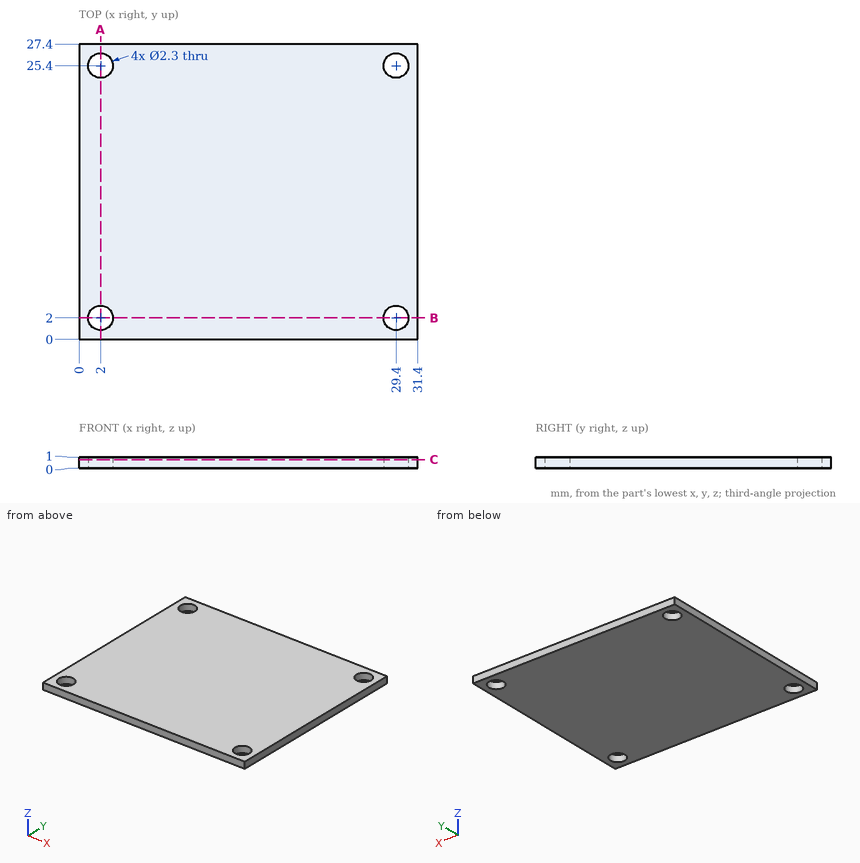
Drawing for the job (mm, zero at the part's lowest x, y, z). Round coordinates to 2 decimals unless told otherwise and drop trailing zeros. Loops run counter-clockwise (first coordinate to the right, second up) from the corner with the lowest first, then second, coordinate; pieces in that order, holes last. Notation, with made-up numbers: (30.25, 69.5) - (73.25, 69.5) arc R18 ccw to (73.25, 92.5) - close; hole circle Ø11 at (-38.5, -32). An arc over 180 degrees is marked (long way). Return JSON: item names as keys, results as strings. Group by question number.
Q1. Band-saw the part on A-A on x = 2. Give the cut face in (y, z).
Q2. Band-saw the part on C-C on z = 0.8. Give the cut face in (x, y), plus the area to 3 significant figures.
Q3. Band-saw the part on B-B on y = 2. Give the cut face in (x, z), plus the area to 3 significant figures.
Q4. Drill centre lines: line 1 along X through (y, z) = (25.4, 0.6); line 2 along Y through (x, z) = (2, 0.5); line 3 along X through (y, z) = (26, 0.25). Where is each one in solid material? Low to high. Write a range as [from, to].
Q5. Flat gauge pins, fed straight in: pin 1 Ø2 at (x, y) = (29.4, 25.4) entering from +Z; pin 2 Ø2.5 at (x, y) = (29.4, 2) entering from +Z. Where does each tip first touch, or does it go through?
Solutions:
{
 "1": {"outline": "(0, 0) - (0.85, 0) - (0.85, 1) - (0, 1) - close; (3.15, 0) - (24.25, 0) - (24.25, 1) - (3.15, 1) - close; (26.55, 0) - (27.4, 0) - (27.4, 1) - (26.55, 1) - close"},
 "2": {"outline": "(0, 0) - (31.4, 0) - (31.4, 27.4) - (0, 27.4) - close; hole circle Ø2.3 at (2, 2); hole circle Ø2.3 at (2, 25.4); hole circle Ø2.3 at (29.4, 2); hole circle Ø2.3 at (29.4, 25.4)", "area": "844 mm^2"},
 "3": {"outline": "(0, 0) - (0.85, 0) - (0.85, 1) - (0, 1) - close; (3.15, 0) - (28.25, 0) - (28.25, 1) - (3.15, 1) - close; (30.55, 0) - (31.4, 0) - (31.4, 1) - (30.55, 1) - close", "area": "26.8 mm^2"},
 "4": {"line 1": "x = [0, 0.85], [3.15, 28.25], [30.55, 31.4]", "line 2": "y = [0, 0.85], [3.15, 24.25], [26.55, 27.4]", "line 3": "x = [0, 1.02], [2.98, 28.42], [30.38, 31.4]"},
 "5": {"pin 1": "passes through", "pin 2": "stops at z = 1"}
}
